Input: dimensioned drawing with shaded views. Units: mm. Origin: part minimum x, y, z. A direction names the side the tool comes from. Round coordinates to 2 decimals unless told otherwise and drop trailing zeros. Order: outer loops, then holes, each group sorted by start corner. A loop starts at its lowest first (then second) coordinate and runs counter-clockwise, first axis right, second up. Notation, with made-up numbers: M 30,-9 L 40,-9 A14 cw 40,-1 Z; hole C 12.5,-36.5 d8. An arc over 180 degrees is marked long. Put each result on its own line as item: value. Start each with the question number.
1) First-contact query: P1, Ø2, axis at x = 13.5, z = 3.5, coming from the -Y side; P2, Ø1, axis at y = 2.5, z = 3, coming from the +X side; P3, Ø2, axis at x = 13.5, z = 2, coming from the +Y side. Flat tips, straight axial feed; report the tip coordinate or a pass-through.
2) Section A-A, the plane z = 0.5. Return loops of the section in (x, y), then the cut area to 3 significant figures.
3) Section B-B, the plane x = 1.5. Return loops of the section in (y, z).
4) Section C-C, the plane y = 17.25. Return loops of the section in (x, z).
5) Material intervals for probe 1 along X at (y, z) = (3, 3.05); probe 2 along Y at (x, z) = (1.5, 0.4); probe 3 along Y at (x, z) = (14.75, 0.65), sorted ascending. Write a range as [from, to].
6) Access query for the marked faces 1, 2 and 3. Directions: +Z, -Z, +X, -X, +Y, -Y. A direction counts if a zero-diameter tool reaches every point of the face in a straight line with its end or side. Return the directions, or none.
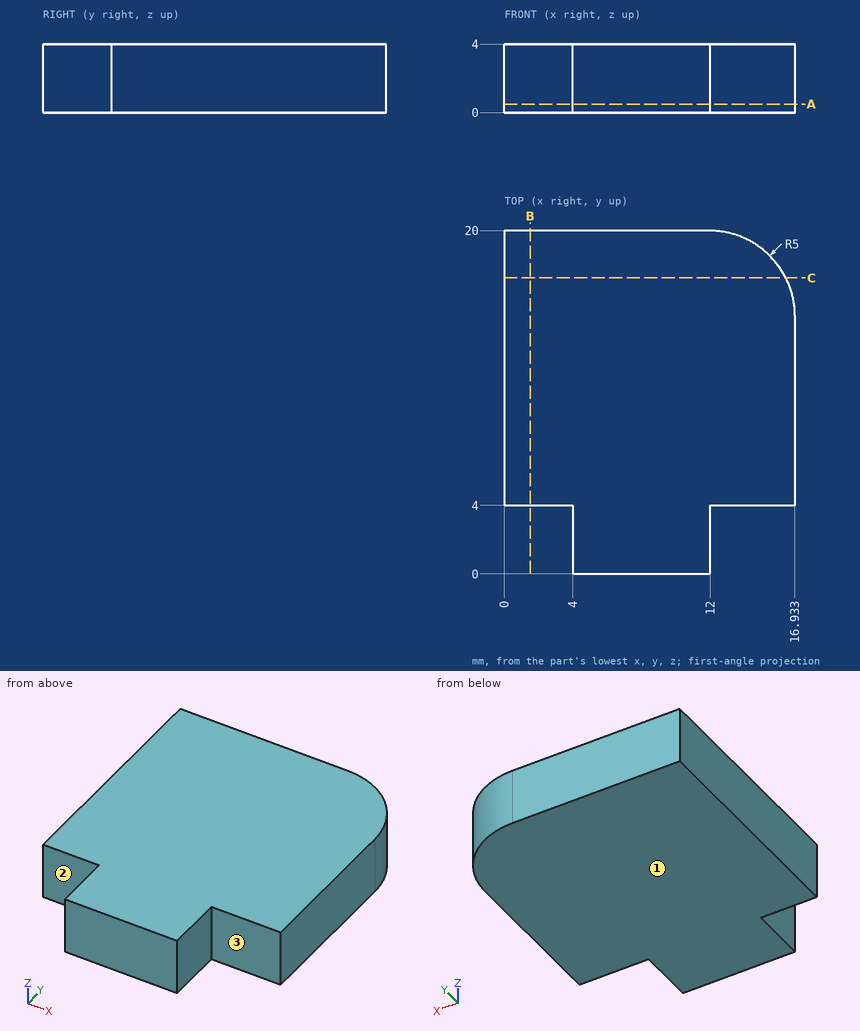
Result sheet:
1. P1: stops at y = 4
1. P2: stops at x = 12
1. P3: stops at y = 19.97
2. outline: M 0,4 L 4,4 L 4,0 L 12,0 L 12,4 L 16.93,4 L 16.93,15 A5 ccw 11.93,20 L 0,20 Z
2. area: 298 mm2
3. outline: M 4,0 L 20,0 L 20,4 L 4,4 Z
4. outline: M 0,0 L 16.4,0 L 16.4,4 L 0,4 Z
5. probe 1: x = [4, 12]
5. probe 2: y = [4, 20]
5. probe 3: y = [4, 19.13]
6. face 1: -Z, +X, -X, +Y, -Y
6. face 2: +Z, -Z, -X, -Y
6. face 3: +Z, -Z, +X, -Y
